Autodesk Inventor part; units mm, degrees
ref_plane "YZ Plane" through (0, 0, 0) normal (1, 0, 0) x (0, 1, 0)
ref_plane "XZ Plane" through (0, 0, 0) normal (0, 1, 0) x (-1, 0, 0)
ref_plane "XY Plane" through (0, 0, 0) normal (0, 0, 1) x (1, 0, 0)
sketch "스케치1" plane through (0, 0, 0) normal (0, 0, 1) x (1, 0, 0)
  line L0 (15, 15) -> (-15, 15)
  line L1 (-15, 15) -> (-15, -15)
  line L2 (-15, -15) -> (15, -15)
  line L3 (15, -15) -> (15, 15)
  circle A0 centre (0, 0) radius 2.5
  circle A1 centre (-10, 10) radius 3
  circle A2 centre (10, 10) radius 3
  circle A3 centre (10, -10) radius 3
  circle A4 centre (-10, -10) radius 3
  line L4 (3.15, 15) -> (-3.15, 15)
  line L5 (-3.15, 15) -> (-3.15, 5)
  line L6 (-3.15, 5) -> (3.15, 5)
  line L7 (3.15, 5) -> (3.15, 15)
  line L8 (-15, -3.15) -> (-5, -3.15)
  line L9 (-5, 3.15) -> (-15, 3.15)
  line L10 (-5, -3.15) -> (-5, 3.15)
  line L11 (-15, 3.15) -> (-15, -3.15)
  line L12 (3.15, -15) -> (3.15, -5)
  line L13 (-3.15, -5) -> (-3.15, -15)
  line L14 (3.15, -5) -> (-3.15, -5)
  line L15 (-3.15, -15) -> (3.15, -15)
  line L16 (15, 3.15) -> (5, 3.15)
  line L17 (5, -3.15) -> (15, -3.15)
  line L18 (5, 3.15) -> (5, -3.15)
  line L19 (15, -3.15) -> (15, 3.15)
  dimension "d0" = 30
  dimension "d1" = 15
  dimension "d2" = 30
  dimension "d3" = 15
  dimension "d4" = 20
  dimension "d5" = 10
  dimension "d6" = 20
  dimension "d7" = 10
  dimension "d8" = 20
  dimension "d9" = 20
  dimension "d10" = 10
  dimension "d11" = 10
  dimension "d12" = 6
  dimension "d13" = 6
  dimension "d14" = 6
  dimension "d15" = 6
  dimension "d16" = 5
  dimension "d17" = 0
  dimension "d18" = 6.3
  dimension "d19" = 3.15
  dimension "d20" = 10
  dimension "d23" = 360
extrude "돌출1" add sketch "스케치1" along normal blind 600 contours L3 L16 L18 L17 L2 L12 L14 L13 L1 L8 L10 L9 L0 L5 L6 L7
equation "\"TransitionRadius\" = BendRadius"
properties part number "3030600"
Part model, mm, in its own coordinate system. A direction names the side the tool comes from. Give positions to 0.01 mm unless a question says otherwise; leave off trailing zeros. Loops run counter-clockwise (first coordinate to the right, second up) from the corner with the lowest first, then second, coordinate; pieces in that order, holes last. Notation, with made-up numbers: M 18,32.25 L 65,32.25 A28 cw 65,50.25 Z; hole C 50.25,-36.5 d3. An arc over 180 degrees is marked long. Put each result on its own line as item: value. Start each with the question number.
1) Saw through at A-A (z = 413.5). List the corners of the cut face in (x, y).
2) 3-axis set-ups, long thin cutter, end or side, ignore diameter. For faces 1 (the flat face through (10, 3.15, 296)), 2 (the flat face through (3.15, 10, 296)), 3 (the flat face through (-10, -3.15, 296)): which of +Z, -Z, +X, -X, +Y, -Y reach the whole face in a straight line?
3) Probe probe 1 along Y at (x, z) = (10, 232); probe 2 along X at (y, z) = (-9.25, 157); probe 3 along X at (y, z) = (-6.25, 158.5). List the from-to ranges inside material, lowest first.
4) Pull direction X, two halves, no side cores. Call faces 4 (the flat face through (15, 9, 296)), 5 (the flat face through (-3.15, -10, 296)), 6 (the flat face through (3.15, -10, 296)), 7 (the flat face through (9, -15, 296)): +X half, -X half, draft (parallel to the pull), parting line (faces both ways), or undercut.
Numbers:
1. outline: M -15,-15 L -3.15,-15 L -3.15,-5 L 3.15,-5 L 3.15,-15 L 15,-15 L 15,-3.15 L 5,-3.15 L 5,3.15 L 15,3.15 L 15,15 L 3.15,15 L 3.15,5 L -3.15,5 L -3.15,15 L -15,15 L -15,3.15 L -5,3.15 L -5,-3.15 L -15,-3.15 Z; hole C -10,-10 d6; hole C -10,10 d6; hole C 0,0 d5; hole C 10,-10 d6; hole C 10,10 d6
2. face 1: +Z, -Z, +X
2. face 2: +Z, -Z, +Y
2. face 3: +Z, -Z, -X
3. probe 1: -15 to -13, -7 to -3.15, 3.15 to 7, 13 to 15
3. probe 2: -15 to -12.9, -7.1 to -3.15, 3.15 to 7.1, 12.9 to 15
3. probe 3: -15 to -3.15, 3.15 to 15
4. face 4: +X half
4. face 5: undercut
4. face 6: undercut
4. face 7: draft
